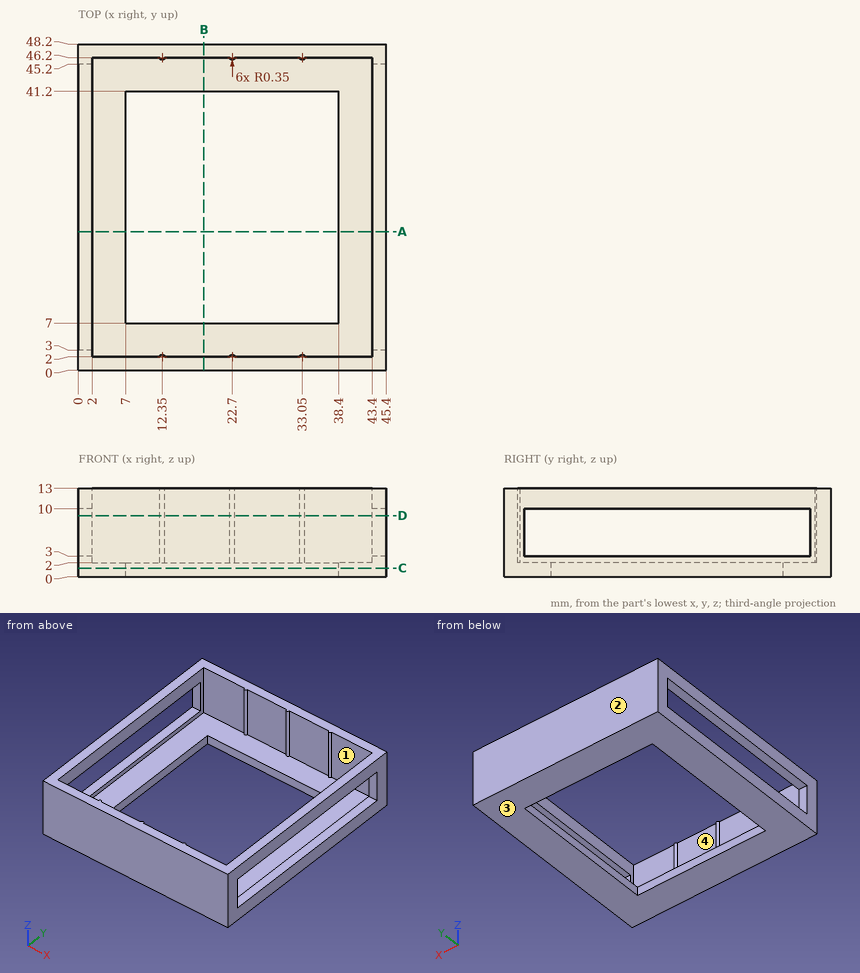
For this review, use the dimensioned drawing (mm, ordinates from the lowest corner) and the shaded views. A direction names the side the tool comes from. Give positions to 0.01 mm unless a question says otherwise; leave off trailing zeros. Loops run counter-clockwise (first coordinate to the right, second up) from the corner with the lowest first, then second, coordinate; pieces in that order, holes last. Notation, with made-up numbers: (13.25, 10.25) - (67.25, 10.25) arc R31 ccw to (67.25, 38.25) - close; hole circle Ø1 at (45, 61.25). An arc over 180 degrees is marked (long way). Write each question's results on one line, items separated by ' | '.
(1) Take a section at D-D (z = 9). Give the boundary of the cut face in (x, y), then the cut area to 3 significant figures.
Conclusion:
outline: (0, 0) - (45.4, 0) - (45.4, 3) - (43.4, 3) - (43.4, 2) - (33.4, 2) arc R0.35 ccw to (32.7, 2) - (23.05, 2) arc R0.35 ccw to (22.35, 2) - (12.7, 2) arc R0.35 ccw to (12, 2) - (2, 2) - (2, 3) - (0, 3) - close; (0, 45.2) - (2, 45.2) - (2, 46.2) - (12, 46.2) arc R0.35 ccw to (12.7, 46.2) - (22.35, 46.2) arc R0.35 ccw to (23.05, 46.2) - (32.7, 46.2) arc R0.35 ccw to (33.4, 46.2) - (43.4, 46.2) - (43.4, 45.2) - (45.4, 45.2) - (45.4, 48.2) - (0, 48.2) - close | area: 191 mm^2
(2) For the marked faces 1 and 2, list the 3-axis set-ups (+Z, -Z, +X, -X, +Y, -Y) from which the entire face can be reached by the end or side of a thin tool; tool diameter is ignored.
Conclusion:
face 1: +Z | face 2: +Z, -Z, +X, -X, +Y
(3) For pin 1 Ø5 at (x, z) = (7, 7) entering from -Y; pin 2 Ø2 at (y, z) = (21.5, 5) entering from +X; pin 3 Ø10 at (x, y) = (10.5, 29.5) entering from +Z, all flat-tipped, find the tip position at first contact; note any pin that passes through.
Conclusion:
pin 1: y = 0 | pin 2: through | pin 3: z = 2
(4) Take a section at B-B (x = 18.5). Give the boundary of the cut face in (y, z).
Conclusion:
outline: (0, 0) - (7, 0) - (7, 2) - (2, 2) - (2, 13) - (0, 13) - close; (41.2, 0) - (48.2, 0) - (48.2, 13) - (46.2, 13) - (46.2, 2) - (41.2, 2) - close
(5) Take a section at C-C (z = 1.25). Give the boundary of the cut face in (x, y).
Conclusion:
outline: (0, 0) - (45.4, 0) - (45.4, 48.2) - (0, 48.2) - close; hole (7, 7) - (38.4, 7) - (38.4, 41.2) - (7, 41.2) - close
(6) For line 1 along Y through (x, z) = (31, 7.5); line 2 along X through (y, z) = (16.5, 11.25); line 3 along X through (y, z) = (15, 1.75), list the stretches that pass through material, from the lowest coordinate up.
Conclusion:
line 1: 0 to 2, 46.2 to 48.2 | line 2: 0 to 2, 43.4 to 45.4 | line 3: 0 to 7, 38.4 to 45.4
(7) Draft analysis for pull direction X (two halves, no side actions). For the marked faces 3 and 4, state which applies: +X half, -X half, draft (parallel to the pull), parting line (faces both ways), or undercut.
Conclusion:
face 3: draft | face 4: undercut
(8) Take a section at A-A (y = 20.5). Give the boundary of the cut face in (x, z).
Conclusion:
outline: (0, 0) - (7, 0) - (7, 2) - (2, 2) - (2, 3) - (0, 3) - close; (0, 10) - (2, 10) - (2, 13) - (0, 13) - close; (38.4, 0) - (45.4, 0) - (45.4, 3) - (43.4, 3) - (43.4, 2) - (38.4, 2) - close; (43.4, 10) - (45.4, 10) - (45.4, 13) - (43.4, 13) - close
